The model under review builds one solid part; all positions refer to its coordinate system, in mm. Face numbers are marked on the shaded views. A direction names the side the tool comes from. Coordinates: 2 decimals unless noted, no trailing zeros. Order: outer loops, then holes, each group sorted by start corner. A loop starts at its lowest first (then second) coordinate and runs counter-clockwise, first axis right, second up. Notation, with made-up numbers: (79.25, -35) - (131.25, -35) arc R21 ccw to (131.25, -28) - close; hole circle Ø11 at (20, 10). An arc over 180 degrees is marked (long way). Answer in a Markdown table with one row per item.
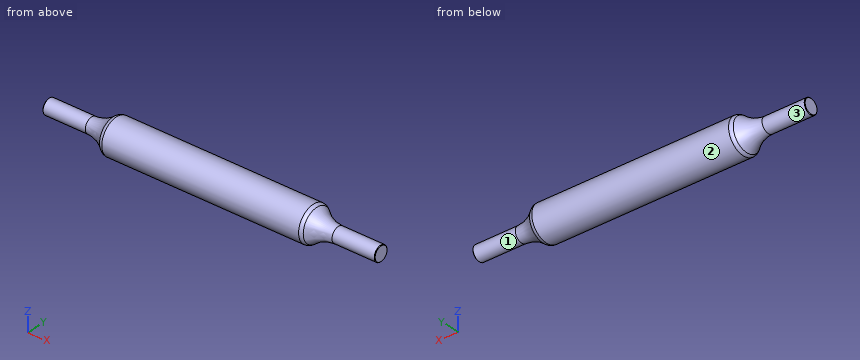
```python
from build123d import *

# Parameters (mm, degrees)
FILLET1_R     = 0.5
CHAMFER1_SIZE = 0.05


with BuildPart() as part:
    # Sketch1 → Revolve1 (revolve)
    with BuildSketch(Plane.XY, mode=Mode.PRIVATE) as revolve1_sk:
        with BuildLine():
            Line((-16.525, 0), (16.525, 0))
            Line((16.525, 0), (16.525, 0.75))
            Line((16.525, 0.75), (12.275, 0.75))
            ThreePointArc((12.275, 0.75), (11.032459759, 1.011033452), (10, 1.75))
            Line((10, 1.75), (-10, 1.75))
            ThreePointArc((-10, 1.75), (-11.032459759, 1.011033452), (-12.275, 0.75))
            Line((-12.275, 0.75), (-16.525, 0.75))
            Line((-16.525, 0.75), (-16.525, 0))
        make_face()
    revolve(revolve1_sk.sketch.rotate(Axis((-16.525, 0, 0), (1, 0, 0)), 180), axis=Axis((-16.525, 0, 0), (1, 0, 0)))

    # Fillet1
    fillet1_edges = [part.edges().sort_by_distance(p)[0] for p in [
        (-10, 1.75, 0),
        (10, 1.75, 0),
    ]]
    fillet(fillet1_edges, radius=FILLET1_R)

    # Chamfer1
    chamfer1_edges = [part.edges().sort_by_distance(p)[0] for p in [
        (-16.525, 0.75, 0),
        (16.525, 0.75, 0),
    ]]
    chamfer(chamfer1_edges, length=CHAMFER1_SIZE)


solid = part.part
```
Item 1: We need section B-B, the plane x = -14. Write out the cut boundary in (y, z).
Check values:
| item | result |
|---|---|
| outline | circle Ø1.5 at (0, 0) |
Item 2: To check wall thickness, follow line 1 (Y direction, x = -1.5, z = 0.25); line 2 (Y direction, x = 3, z = -1.05); line 3 (Z direction, x = -8, y = -1.25). State the ranges of each line that lie inside material, in increasing order. Write a range as from..to.
Check values:
| item | result |
|---|---|
| line 1 | -1.73..1.73 |
| line 2 | -1.4..1.4 |
| line 3 | -1.22..1.22 |
Item 3: Tool access review of the marked faces 1, 2 and 3: name each direction out of +Z, -Z, +X, -X, +Y, -Y from which nothing blocks a thin tool from reaching the whole face with its end or side.
Check values:
| item | result |
|---|---|
| face 1 | +X |
| face 2 | +X, -X |
| face 3 | -X |
Item 4: We need section A-A, the plane x = 7. Write out the cut boundary in (y, z), then the cut area to 3 significant figures.
Check values:
| item | result |
|---|---|
| outline | circle Ø3.5 at (0, 0) |
| area | 9.62 mm^2 |
Item 5: Clearance check with flat-ended pins moving along their axes: pin 1 Ø1.5 at (x, y) = (2.5, -1.5) entering from -Z; pin 2 Ø1.5 at (x, y) = (3, 1) entering from -Z. State where each tip first meets the part, or that it passes through.
Check values:
| item | result |
|---|---|
| pin 1 | z = -1.58 |
| pin 2 | z = -1.73 |
